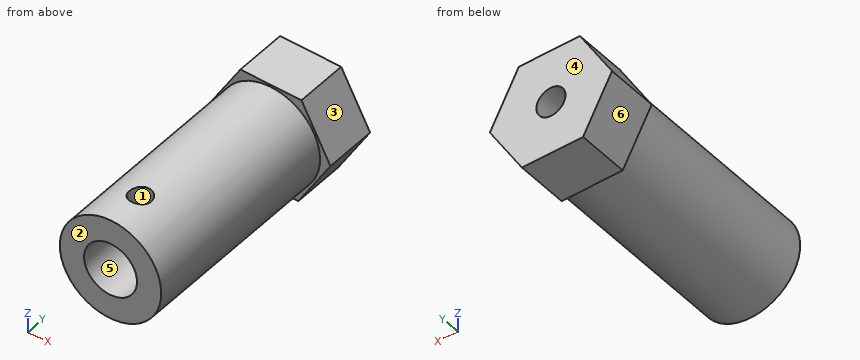
from build123d import *

# Parameters (mm, degrees)
SKETCH_1_R             = 5.75
SKETCH_1_R_2           = 3
EXTRUDE_1_DEPTH        = 24
HOLE_WIZARD_M3_1_D     = 2.5
HOLE_WIZARD_M3_1_DEPTH = 7.748924226
HOLE_WIZARD_M3_1_TIP   = 0.751075774
EXTRUDE_2_DEPTH        = 6
HOLE_WIZARD_M4_1_D     = 3.3


with BuildPart() as part:
    # 草图1 → 凸台-拉伸1 (new body)
    with BuildSketch(Plane(origin=(0, 0, 0), x_dir=(1, 0, 0), z_dir=(0, 1, 0))):
        with Locations(Location((0, 0, 0), (0, 0, 270))):
            Circle(SKETCH_1_R)
        with Locations(Location((0, 0, 0), (0, 0, 270))):
            Circle(SKETCH_1_R_2, mode=Mode.SUBTRACT)
    extrude(amount=EXTRUDE_1_DEPTH)

    # M3 螺纹孔1
    with Locations(Plane.XY.offset(5.75)):
        with Locations((0, 4.5)):
            Hole(HOLE_WIZARD_M3_1_D / 2, depth=HOLE_WIZARD_M3_1_DEPTH)
            with Locations((0, 0, -(HOLE_WIZARD_M3_1_DEPTH + HOLE_WIZARD_M3_1_TIP / 2))):  # 118° drill point
                Cone(0, HOLE_WIZARD_M3_1_D / 2, HOLE_WIZARD_M3_1_TIP, mode=Mode.SUBTRACT)

    # 草图11 → 凸台-拉伸2 (add)
    with BuildSketch(Plane(origin=(0, 24, 0), x_dir=(1, 0, 0), z_dir=(0, 1, 0))):
        Polygon((6.925181727, 0.204592398), (3.28540865, 6.0996795), (-3.639773077, 5.895087103), (-6.925181727, -0.204592398), (-3.28540865, -6.0996795), (3.639773077, -5.895087103), align=None)
    extrude(amount=EXTRUDE_2_DEPTH)

    # M4 螺纹孔的螺纹孔钻头1 (through all)
    with Locations(Plane(origin=(0, 30, 0), x_dir=(1, 0, 0), z_dir=(0, 1, 0))):
        with Locations((0, 0)):
            Hole(HOLE_WIZARD_M4_1_D / 2)


solid = part.part
Check sheet for the modelled part. Datum: model origin and axes. Units: mm. Face numbers are marked on the shaded views. A direction names the side the tool comes from. Round coordinates to 2 decimals unless told otherwise and drop trailing zeros. Loops run counter-clockwise (first coordinate to the right, second up) from the corner with the lowest first, then second, coordinate; pieces in that order, holes last. Notation, with made-up numbers: (62, 21.25) -> (118, 21.25) arc R15 ccw to (118, 30.25) -> close; hole circle Ø10 at (-5.5, -29.5). An arc over 180 degrees is marked (long way). Put each result on its own line as item: value. Start each with the question number.
1. Gauge pin test, flat ends, axial feed: pin 1 (4 mm diameter, centred on y = 22.5, z = 2.5, fed in from +X); pin 2 (8 mm diameter, centred on x = -2.5, y = 11.5, fed in from -Z); pin 3 (2 mm diameter, centred on x = -1, z = 0, fed in from -Y); pin 4 (3 mm diameter, centred on x = 0, z = 0, fed in from -Y). Record the tip position at first contact, or that the pin passes through.
2. Section check D-D (x = 0). Enter the section's corners in (y, z).
3. Access from +Z, -Z, +X, -X, +Y, -Y to the whole of each face (thin tool, end or side, straight path). Record for the marked faces 5 and 6.
4. Section check A-A (y = 26). Enter the section's corners in (x, z), plus the area to 3 significant figures.
5. Section check C-C (z = 5). Enter the section's corners in (x, y).
6. Section check B-B (z = -0.5). Enter the section's corners in (x, y).
7. Scan lines: probe 1 along Y at (x, z) = (0, 4); probe 2 along X at (y, z) = (15, 0); probe 3 along X at (y, z) = (27, -0.75). Record each from-to range of solid material in increasing order.
8. Draft check along Y on the marked faces 1, 2, 3 and 4. Enter one of: +Y half, -Y half, draft (parallel to the pull), parting line (faces both ways), or undercut.
Findings:
1. pin 1: stops at x = 6.18
1. pin 2: stops at z = -5.75
1. pin 3: stops at y = 24
1. pin 4: passes through
2. outline: (0, -5.75) -> (24, -5.75) -> (24, -6) -> (30, -6) -> (30, -1.65) -> (24, -1.65) -> (24, -3) -> (0, -3) -> close; (0, 3) -> (3.25, 3) -> (3.25, 5.75) -> (0, 5.75) -> close; (5.75, 3) -> (24, 3) -> (24, 1.65) -> (30, 1.65) -> (30, 6) -> (24, 6) -> (24, 5.75) -> (5.75, 5.75) -> close
3. face 5: -Y
3. face 6: -Z, -X, +Y, -Y
4. outline: (-6.93, 0.2) -> (-3.64, -5.9) -> (3.29, -6.1) -> (6.93, -0.2) -> (3.64, 5.9) -> (-3.29, 6.1) -> close; hole circle Ø3.3 at (0, 0)
4. area: 116 mm^2
5. outline: (-3.96, 24) -> (-2.84, 24) -> (-2.84, 0) -> (2.84, 0) -> (2.84, 24) -> (4.12, 24) -> (4.12, 30) -> (-3.96, 30) -> close; hole circle Ø2.5 at (0, 4.5)
6. outline: (-6.55, 24) -> (-5.73, 24) -> (-5.73, 0) -> (-2.96, 0) -> (-2.96, 24) -> (-1.57, 24) -> (-1.57, 30) -> (-6.55, 30) -> close; (1.57, 24) -> (2.96, 24) -> (2.96, 0) -> (5.73, 0) -> (5.73, 24) -> (6.74, 24) -> (6.74, 30) -> (1.57, 30) -> close
7. probe 1: y = 0 to 3.25, 5.75 to 30
7. probe 2: x = -5.75 to -3, 3 to 5.75
7. probe 3: x = -6.41 to -1.47, 1.47 to 6.59
8. face 1: undercut
8. face 2: -Y half
8. face 3: draft
8. face 4: +Y half
